from build123d import *

# Parameters (mm, degrees)
SKETCH1_W           = 42
SKETCH1_H           = 132
BOSS_EXTRUDE1_DEPTH = 3
SKETCH2_R           = 2.5
CUT_EXTRUDE1_DEPTH  = 2
SKETCH3_R           = 1.5
CUT_EXTRUDE2_DEPTH  = 70.289248805
CUT_EXTRUDE3_DEPTH  = 70.32532005


with BuildPart() as part:
    # Sketch1 → Boss-Extrude1 (new body)
    with BuildSketch(Plane(origin=(0, 0, 0), x_dir=(1, 0, 0), z_dir=(0, 1, 0))):
        Rectangle(SKETCH1_W, SKETCH1_H)
    extrude(amount=BOSS_EXTRUDE1_DEPTH)

    # Sketch2 → Cut-Extrude1 (cut)
    with BuildSketch(Plane(origin=(0, 3, 0), x_dir=(1, 0, 0), z_dir=(0, 1, 0))):
        with Locations(Location((-16.5, 61.5, 0), (0, 0, 270))):
            Circle(SKETCH2_R)
        with Locations(Location((16.5, 61.5, 0), (0, 0, 270))):
            Circle(SKETCH2_R)
        with Locations(Location((16.5, -61.5, 0), (0, 0, 270))):
            Circle(SKETCH2_R)
        with Locations(Location((-16.5, -61.5, 0), (0, 0, 270))):
            Circle(SKETCH2_R)
    extrude(amount=-CUT_EXTRUDE1_DEPTH, mode=Mode.SUBTRACT)

    # Sketch3 → Cut-Extrude2 (cut, through all)
    with BuildSketch(Plane(origin=(0, 1, 0), x_dir=(1, 0, 0), z_dir=(0, 1, 0))):
        with Locations(Location((-16.5, 61.5, 0), (0, 0, 270))):
            Circle(SKETCH3_R)
        with Locations(Location((16.5, 61.5, 0), (0, 0, 270))):
            Circle(SKETCH3_R)
        with Locations(Location((16.5, -61.5, 0), (0, 0, 270))):
            Circle(SKETCH3_R)
        with Locations(Location((-16.5, -61.5, 0), (0, 0, 270))):
            Circle(SKETCH3_R)
    extrude(amount=-CUT_EXTRUDE2_DEPTH, mode=Mode.SUBTRACT)

    # Sketch4 → Cut-Extrude3 (cut, through all)
    with BuildSketch(Plane(origin=(0, 3, 0), x_dir=(1, 0, 0), z_dir=(0, 1, 0))):
        Polygon((21, -353.041513135), (21, -66), (21, 66), (19.84024034, 66), (19.84024034, -66), (19.84024034, -353.041513135), (19.84024034, -927.124539404), (21, -927.124539404), align=None)
    extrude(amount=-CUT_EXTRUDE3_DEPTH, mode=Mode.SUBTRACT)


solid = part.part
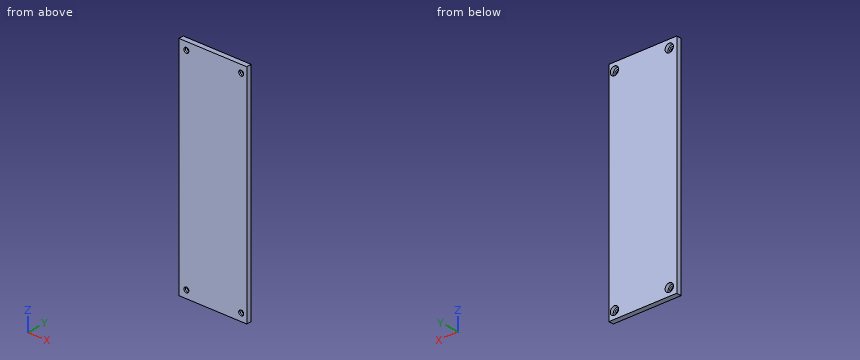
The listing builds one solid part. Answer for the finished solid, in the listing's coordinates (mm). Give positions to 0.01 mm unless a question says otherwise; leave off trailing zeros. Write each loop counter-clockwise with the first axis right and the second up, starting at its lowest first coordinate (ties: lowest second). Pieces come first, ordered by that corner, then holes.
1) Section B-B (x = 16.5) is taken. Write down the section's boundary in (y, z), and give its area (3 significant figures).
2) Find the intervals of material crossed by L1, parallel to X at y = 0.5, z = 61.5; L2, parallel to X at y = 1.5, z = 61.5; L3, parallel to Z at x = -16, y = 1.25, in increasing order.
3) Section A-A (z = -61.5) is taken. Write down the section's boundary in (x, y).
4) Given P1, Ø3.5, axis at x = -16.5, z = -61.5, coming from the +Y side, flat-ended and moving along its own axis, determine where the tip first touches the part or whether it passes through.
Response:
1. outline: (0, -66) - (3, -66) - (3, -64) - (1, -64) - (1, -63) - (0, -63) - close; (0, -60) - (1, -60) - (1, -59) - (3, -59) - (3, 59) - (1, 59) - (1, 60) - (0, 60) - close; (0, 63) - (1, 63) - (1, 64) - (3, 64) - (3, 66) - (0, 66) - close
1. area: 370 mm2
2. L1: x = -21 to -18, -15 to 15, 18 to 19.84
2. L2: x = -21 to -19, -14 to 14, 19 to 19.84
2. L3: z = -66 to -63.95, -59.05 to 59.05, 63.95 to 66
3. outline: (-21, 0) - (-18, 0) - (-18, 1) - (-19, 1) - (-19, 3) - (-21, 3) - close; (-15, 0) - (15, 0) - (15, 1) - (14, 1) - (14, 3) - (-14, 3) - (-14, 1) - (-15, 1) - close; (18, 0) - (19.84, 0) - (19.84, 3) - (19, 3) - (19, 1) - (18, 1) - close
4. P1: stops at y = 1
